Geometry check sheet. Reference: the model listing, model coordinates, mm. A direction names the side the tool comes from. Give positions to 0.01 mm unless a question says otherwise; leave off trailing zeros. Loops run counter-clockwise (first coordinate to the right, second up) from the corner with the lowest first, then second, coordinate; pieces in that order, holes last.
Autodesk Inventor part; units mm, degrees
ref_plane "Work Plane1" through (50.664548, -102.160446, 0.616313) normal (0, -0.9659258, -0.258819) x (1, 0, 0)
ref_plane "YZ Plane" through (0, 0, 0) normal (1, 0, 0) x (0, 1, 0)
ref_plane "XZ Plane" through (0, 0, 0) normal (0, 1, 0) x (-1, 0, 0)
sketch "Sketch1" plane through (0, 0, 0) normal (0, 0, 1) x (1, 0, 0)
  line L0 (-10.454202, 14.601943) -> (210.208298, 14.601943)
  line L1 (216.558298, 8.251943) -> (216.558298, -98.110557)
  line L2 (210.208298, -104.460557) -> (-10.454202, -104.460557)
  line L3 (-16.804202, -98.110557) -> (-16.804202, 8.251943)
  line L4 (99.877048, 12.220693) -> (-10.454202, 12.220693)
  line L5 (-14.422952, 8.251943) -> (-14.422952, -44.929307)
  line L6 (99.877048, 12.220693) -> (210.208298, 12.220693)
  line L7 (214.177048, 8.251943) -> (214.177048, -44.929307)
  line L8 (99.877048, -102.079307) -> (210.208298, -102.079307)
  line L9 (214.177048, -98.110557) -> (214.177048, -44.929307)
  line L10 (99.877048, -102.079307) -> (-10.454202, -102.079307)
  line L11 (-14.422952, -98.110557) -> (-14.422952, -44.929307)
  arc A0 (-10.454202, 14.601943) -> (-16.804202, 8.251943) centre (-10.454202, 8.251943) ccw
  arc A1 (216.558298, 8.251943) -> (210.208298, 14.601943) centre (210.208298, 8.251943) ccw
  arc A2 (210.208298, -104.460557) -> (216.558298, -98.110557) centre (210.208298, -98.110557) ccw
  arc A3 (-16.804202, -98.110557) -> (-10.454202, -104.460557) centre (-10.454202, -98.110557) ccw
  arc A4 (-10.454202, 12.220693) -> (-14.422952, 8.251943) centre (-10.454202, 8.251943) ccw
  arc A5 (214.177048, 8.251943) -> (210.208298, 12.220693) centre (210.208298, 8.251943) ccw
  arc A6 (210.208298, -102.079307) -> (214.177048, -98.110557) centre (210.208298, -98.110557) ccw
  arc A7 (-14.422952, -98.110557) -> (-10.454202, -102.079307) centre (-10.454202, -98.110557) ccw
  point P0 (0, 0)
  point P1 (-16.804202, 14.601943)
  point P2 (216.558298, -104.460557)
  point P3 (216.558298, 14.601943)
  point P4 (-16.804202, -104.460557)
  dimension "d0" = 233.3625
  dimension "d1" = 119.0625
  dimension "d9" = 6.35
  dimension "d10" = 3.96875
extrude "Extrusion1" add sketch "Sketch1" along normal blind 2.38125 contours L0 A1 L1 A2 L2 A3 L3 A0 | L6 A5 L7 L9 A6 L8 L10 A7 L11 L5 A4 L4
sketch "Sketch2" plane through (0, 0, 2.38125) normal (0, 0, 1) x (1, 0, 0)
  line L0 (210.208298, 14.601943) -> (-10.454202, 14.601943)
  arc A0 (-10.454202, 14.601943) -> (-16.804202, 8.251943) centre (-10.454202, 8.251943) ccw
  line L1 (-16.804202, 8.251943) -> (-16.804202, -98.110557)
  arc A1 (-16.804202, -98.110557) -> (-10.454202, -104.460557) centre (-10.454202, -98.110557) ccw
  line L2 (-10.454202, -104.460557) -> (210.208298, -104.460557)
  arc A2 (210.208298, -104.460557) -> (216.558298, -98.110557) centre (210.208298, -98.110557) ccw
  line L3 (216.558298, -98.110557) -> (216.558298, 8.251943)
  arc A3 (216.558298, 8.251943) -> (210.208298, 14.601943) centre (210.208298, 8.251943) ccw
  line L4 (99.877048, 12.220693) -> (-10.454202, 12.220693)
  line L5 (-14.422952, 8.251943) -> (-14.422952, -44.929307)
  line L6 (99.877048, -102.079307) -> (-10.454202, -102.079307)
  line L7 (-14.422952, -98.110557) -> (-14.422952, -44.929307)
  line L8 (99.877048, -102.079307) -> (210.208298, -102.079307)
  line L9 (214.177048, -98.110557) -> (214.177048, -44.929307)
  line L10 (99.877048, 12.220693) -> (210.208298, 12.220693)
  line L11 (214.177048, 8.251943) -> (214.177048, -44.929307)
  arc A4 (-10.454202, 12.220693) -> (-14.422952, 8.251943) centre (-10.454202, 8.251943) ccw
  arc A5 (214.177048, 8.251943) -> (210.208298, 12.220693) centre (210.208298, 8.251943) ccw
  arc A6 (210.208298, -102.079307) -> (214.177048, -98.110557) centre (210.208298, -98.110557) ccw
  arc A7 (-14.422952, -98.110557) -> (-10.454202, -102.079307) centre (-10.454202, -98.110557) ccw
  point P0 (0, 0)
  dimension "d15" = 3.96875
extrude "Extrusion2" add sketch "Sketch2" along normal blind 2.38125
sketch "Sketch3" plane through (0, 0, 4.7625) normal (0, 0, 1) x (1, 0, 0)
  arc A0 (-10.454202, 12.220693) -> (-14.422952, 8.251943) centre (-10.454202, 8.251943) ccw
  line L0 (-10.454202, 12.220693) -> (210.208298, 12.220693)
  arc A1 (214.177048, 8.251943) -> (210.208298, 12.220693) centre (210.208298, 8.251943) ccw
  line L1 (214.177048, 8.251943) -> (214.177048, -98.110557)
  arc A2 (210.208298, -102.079307) -> (214.177048, -98.110557) centre (210.208298, -98.110557) ccw
  line L2 (210.208298, -102.079307) -> (-10.454202, -102.079307)
  arc A3 (-14.422952, -98.110557) -> (-10.454202, -102.079307) centre (-10.454202, -98.110557) ccw
  line L3 (-14.422952, -98.110557) -> (-14.422952, 8.251943)
  line L4 (210.208298, 14.601943) -> (-10.454202, 14.601943)
  arc A4 (-10.454202, 14.601943) -> (-16.804202, 8.251943) centre (-10.454202, 8.251943) ccw
  line L5 (-16.804202, 8.251943) -> (-16.804202, -98.110557)
  arc A5 (-16.804202, -98.110557) -> (-10.454202, -104.460557) centre (-10.454202, -98.110557) ccw
  line L6 (-10.454202, -104.460557) -> (210.208298, -104.460557)
  arc A6 (210.208298, -104.460557) -> (216.558298, -98.110557) centre (210.208298, -98.110557) ccw
  line L7 (216.558298, -98.110557) -> (216.558298, 8.251943)
  arc A7 (216.558298, 8.251943) -> (210.208298, 14.601943) centre (210.208298, 8.251943) ccw
  line L8 (214.177048, -44.929307) -> (214.177048, -41.754307)
  line L9 (214.177048, -41.754307) -> (216.558298, -41.754307)
  line L10 (216.558298, -41.754307) -> (216.558298, -44.929307)
  line L11 (216.558298, -44.929307) -> (216.558298, -48.104307)
  line L12 (216.558298, -48.104307) -> (214.177048, -48.104307)
  line L13 (214.177048, -48.104307) -> (214.177048, -44.929307)
  line L14 (-14.422952, -44.929307) -> (-14.422952, -41.754307)
  line L15 (-14.422952, -41.754307) -> (-16.804202, -41.754307)
  line L16 (-16.804202, -41.754307) -> (-16.804202, -44.929307)
  line L17 (-16.804202, -44.929307) -> (-16.804202, -48.104307)
  line L18 (-16.804202, -48.104307) -> (-14.422952, -48.104307)
  line L19 (-14.422952, -48.104307) -> (-14.422952, -44.929307)
  point P0 (0, 0)
  dimension "d18" = 3.175
  dimension "d19" = 3.175
  dimension "d20" = 3.175
  dimension "d21" = 3.175
extrude "Extrusion3" add sketch "Sketch3" along normal blind 10.31875 contours A0 L3 L15 L5 A4 L4 A7 L7 L9 L1 A1 L0 | L3 A3 L2 A2 L1 L12 L7 A6 L6 A5 L5 L18
sketch "Sketch4" plane through (0, 0, 15.08125) normal (0, 0, 1) x (1, 0, 0)
  line L0 (214.177048, -41.754307) -> (216.558298, -41.754307)
  line L1 (216.558298, -41.754307) -> (216.558298, -48.104307)
  line L2 (216.558298, -48.104307) -> (214.177048, -48.104307)
  line L3 (214.177048, -48.104307) -> (214.177048, -41.754307)
  line L4 (-16.804202, -41.754307) -> (-14.422952, -41.754307)
  line L5 (-14.422952, -41.754307) -> (-14.422952, -48.104307)
  line L6 (-14.422952, -48.104307) -> (-16.804202, -48.104307)
  line L7 (-16.804202, -48.104307) -> (-16.804202, -41.754307)
  point P0 (0, 0)
  dimension "d24" = 2.38125
  dimension "d25" = 6.35
  dimension "d26" = 2.38125
  dimension "d27" = 6.35
extrude "Extrusion4" add sketch "Sketch4" against normal blind 7.9375
sketch "Sketch5" plane through (0, 0, 0) normal (0, 0, -1) x (-1, 0, 0)
  arc A0 (-210.208298, 14.601943) -> (-216.558298, 8.251943) centre (-210.208298, 8.251943) ccw
  line L0 (-210.208298, 8.251943) -> (-99.877048, 8.251943)
  line L1 (-99.877048, 8.251943) -> (-99.877048, -44.929307)
  line L2 (-99.877048, -44.929307) -> (-210.208298, -44.929307)
  line L3 (-210.208298, -44.929307) -> (-210.208298, 8.251943)
  point P0 (0, 0)
hole "Hole1" at (99.877048, -44.929307, 0) direction (0, 0, 1) diameter 19.05 end through all
sketch "Sketch7" plane through (-10.454202, -104.460557, 0) normal (0, -1, 0) x (1, 0, 0)
  line L0 (220.6625, 0) -> (0, 0)
  line L1 (0, 15.08125) -> (220.6625, 15.08125)
  line L2 (61.11875, 15.08125) -> (61.11875, 0)
  line L3 (159.54375, 15.08125) -> (159.54375, 0)
  line L4 (61.11875, 15.08125) -> (159.54375, 15.08125)
  line L5 (159.54375, 0) -> (61.11875, 0)
  point P0 (10.454202, 0)
extrude "Extrusion5" add sketch "Sketch7" along normal blind 25.4
sketch "Sketch8" plane through (149.089548, -104.460557, 15.08125) normal (1, 0, 0) x (0, 0, -1)
  line L0 (15.08125, 0) -> (-19.502452, -9.266675)
  line L1 (15.08125, 0) -> (50.884933, 0) construction
  point P0 (15.08125, 104.460557)
  dimension "d41" = 165
split body "Split1" sketch "Sketch8" result one side removed curves L0 removed pieces at (116.281215, -121.39389, 0.5)
ref_plane "Work Plane1" through (50.664548, -102.160446, 0.616313) normal (0, -0.9659258, -0.258819) x (1, 0, 0)
sketch "Sketch10" plane through (0, 0, 15.08125) normal (0, 0, 1) x (1, 0, 0)
  line L0 (99.877048, -104.460557) -> (111.307048, -104.460557)
  line L1 (111.307048, -104.460557) -> (111.307048, -108.501565)
  line L2 (99.877048, -104.460557) -> (88.447048, -104.460557)
  line L3 (88.447048, -104.460557) -> (88.447048, -108.501565)
  line L4 (88.447048, -108.501565) -> (111.307048, -108.501565)
  point P0 (0, 0)
  dimension "d43" = 11.43
  dimension "d44" = 11.43
split body "Split2" sketch "Sketch10" result one side removed curves L4 L1 L0 L2 L3 removed pieces at (99.877048, -106.671599, 10.183576)
sketch "Sketch13" plane through (50.664548, -102.160446, 0.616313) normal (0, -0.9659258, -0.258819) x (1, 0, 0)
  line L0 (37.7825, 0) -> (37.7825, 15.613259)
  line L1 (0, 15.613259) -> (37.7825, 15.613259)
  line L2 (0, 0) -> (0, 15.613259)
  line L3 (37.7825, 0) -> (0, 0)
  line L4 (60.6425, 15.613259) -> (60.6425, 0)
  line L5 (98.425, 0) -> (60.6425, 0)
  line L6 (98.425, 15.613259) -> (98.425, 0)
  line L7 (60.6425, 15.613259) -> (98.425, 15.613259)
  line L8 (0, 15.613259) -> (98.425, 15.613259)
  line L9 (49.2125, 15.613259) -> (49.2125, 0)
  line L10 (49.2125, 7.806629) -> (32.8295, 7.806629)
  line L11 (49.2125, 7.806629) -> (65.5955, 7.806629)
  line L12 (65.5955, 7.806629) -> (80.0735, 7.806629)
  line L13 (32.8295, 7.806629) -> (18.3515, 7.806629)
  point P0 (-50.664548, -27.036381)
  dimension "d45" = 16.383
  dimension "d46" = 16.383
  dimension "d47" = 14.478
  dimension "d48" = 14.478
hole "Hole2" at (69.016048, -104.18095, 8.156938) at (116.260048, -104.18095, 8.156938) at (83.494048, -104.18095, 8.156938) at (130.738048, -104.18095, 8.156938) direction (0, 0.9659258, 0.258819) diameter 6.35 end through all
sketch "Sketch14" plane through (50.664548, -102.160446, 0.616313) normal (0, -0.9659258, -0.258819) x (1, 0, 0)
  line L0 (37.7825, 0) -> (37.7825, 15.613259)
  line L1 (0, 15.613259) -> (37.7825, 15.613259)
  line L2 (0, 0) -> (0, 15.613259)
  line L3 (37.7825, 0) -> (0, 0)
  line L4 (60.6425, 15.613259) -> (60.6425, 0)
  line L5 (98.425, 0) -> (60.6425, 0)
  line L6 (98.425, 15.613259) -> (98.425, 0)
  line L7 (60.6425, 15.613259) -> (98.425, 15.613259)
  line L8 (0, 15.613259) -> (98.425, 15.613259)
  line L9 (49.2125, 15.613259) -> (49.2125, 0)
  line L10 (49.2125, 7.806629) -> (65.5955, 7.806629)
  line L11 (65.5955, 7.806629) -> (80.0735, 7.806629)
  line L12 (49.2125, 7.806629) -> (32.8295, 7.806629)
  line L13 (32.8295, 7.806629) -> (18.3515, 7.806629)
  point P0 (-50.664548, -27.036381)
  dimension "d56" = 16.383
  dimension "d57" = 14.478
  dimension "d58" = 16.383
  dimension "d59" = 14.478
hole "Hole3" at (69.016048, -104.18095, 8.156938) at (83.494048, -104.18095, 8.156938) at (116.260048, -104.18095, 8.156938) at (130.738048, -104.18095, 8.156938) direction (0, -0.9659258, -0.258819) diameter 3.175 end through all
sketch "Sketch15" plane through (0, 0, 4.7625) normal (0, 0, 1) x (1, 0, 0)
  line L0 (216.558298, -41.754307) -> (214.177048, -41.754307)
  line L1 (214.177048, -41.754307) -> (214.177048, -48.104307)
  line L2 (216.558298, -41.754307) -> (214.177048, -41.754307)
  line L3 (214.177048, -41.754307) -> (214.177048, -48.104307)
  line L4 (214.177048, -48.104307) -> (216.558298, -48.104307)
  line L5 (216.558298, -48.104307) -> (216.558298, -41.754307)
  point P0 (0, 0)
extrude "Extrusion6" add sketch "Sketch15" along normal blind 2.3876
sketch "Sketch16" plane through (0, 0, 4.7625) normal (0, 0, 1) x (1, 0, 0)
  line L0 (-14.422952, -41.754307) -> (-16.804202, -41.754307)
  line L1 (-16.804202, -41.754307) -> (-16.804202, -48.104307)
  line L2 (-14.422952, -41.754307) -> (-16.804202, -41.754307)
  line L3 (-16.804202, -41.754307) -> (-16.804202, -48.104307)
  line L4 (-16.804202, -48.104307) -> (-14.422952, -48.104307)
  line L5 (-14.422952, -48.104307) -> (-14.422952, -41.754307)
  point P0 (0, 0)
extrude "Extrusion7" add sketch "Sketch16" along normal blind 2.3876
sketch "Sketch17" plane through (0, 0, 0) normal (0, 0, -1) x (-1, 0, 0)
  arc A0 (10.454202, -104.460557) -> (16.804202, -98.110557) centre (10.454202, -98.110557) ccw
  arc A1 (16.804202, 8.251943) -> (10.454202, 14.601943) centre (10.454202, 8.251943) ccw
  arc A2 (-210.208298, 14.601943) -> (-216.558298, 8.251943) centre (-210.208298, 8.251943) ccw
  arc A3 (-216.558298, -98.110557) -> (-210.208298, -104.460557) centre (-210.208298, -98.110557) ccw
  point P0 (0, 0)
hole "Hole4" at (210.208298, 8.251943, 0) at (-10.454202, 8.251943, 0) at (-10.454202, -98.110557, 0) at (210.208298, -98.110557, 0) direction (0, 0, 1) diameter 3.175 end through all
properties part number "Master Tablet Enclosure"
1) Sectioned sample at A-A on x = 16.5. Enter the section's corners in (y, z).
2) Sectioned sample at C-C on y = -39.5. Enter the section's corners in (x, z).
3) Depth check by flat-ended pin: P1, Ø1, axis at x = 38, y = -61, coming from the +Z side; P2, Ø1.5, axis at x = 48.5, z = 7.5, coming from the -Y side; P3, Ø2.5, axis at x = 210.21, y = 8.25, coming from the +Z side; P4, Ø2, axis at y = -106.5, z = 5, coming from the +X side. Enter the tip coordinate at first touch or a pass-through.
4) Sectioned sample at D-D on y = -52. Enter the section's corners in (x, z).
5) Tool access check on faces 5 (the flat face through (20, -104.461, 7)), 6 (the flat face through (132.1, -103.83, 6.84)), 7 (the flat face through (149.09, -106, 9)), 8 (the flat face through (88.447, -106, 11)). Record the directions out of +Z, -Z, +X, -X, +Y, -Y that give a thin tool (end or side, any length) a straight path to the whole face; none if there is none.
6) Scan lines: line 1 along Y through (x, z) = (151.5, 11.5); line 2 along X through (y, z) = (-79, 3.75); line 3 along Z through (x, y) = (73, -36). Record each from-to range of solid material in increasing order.
7) Mould release check, pull along Y, two halves, no side actions. Record for faces 1 (the flat face through (179, -104.461, 7)), 2 (the flat face through (98, -57, 2.381)), 3 (the cylindrical face through (-13.23, -100.948, 8.642)), 4 (the flat face through (-16.804, -44, 7)): +Y half, -Y half, draft (parallel to the pull), parting line (faces both ways), or undercut.
8) Sectioned sample at B-B on y = -27. Enter the section's corners in (x, z), plus the area to 3 significant figures.
Determined:
1. outline: (-104.46, 0) - (14.6, 0) - (14.6, 15.08) - (12.22, 15.08) - (12.22, 2.38) - (-102.08, 2.38) - (-102.08, 15.08) - (-104.46, 15.08) - close
2. outline: (-16.8, 0) - (92.05, 0) - (92.05, 2.38) - (-14.42, 2.38) - (-14.42, 15.08) - (-16.8, 15.08) - close; (107.7, 0) - (216.56, 0) - (216.56, 15.08) - (214.18, 15.08) - (214.18, 2.38) - (107.7, 2.38) - close
3. P1: stops at z = 2.38
3. P2: stops at y = -104.46
3. P3: passes through
3. P4: stops at x = 149.09
4. outline: (-16.8, 0) - (93.49, 0) - (93.49, 2.38) - (-14.42, 2.38) - (-14.42, 15.08) - (-16.8, 15.08) - close; (106.26, 0) - (216.56, 0) - (216.56, 15.08) - (214.18, 15.08) - (214.18, 2.38) - (106.26, 2.38) - close
5. face 5: +Z, -Z, -X, -Y
5. face 6: none
5. face 7: +Z, -Z, +X, -Y
5. face 8: +Z, -Z, -Y
6. line 1: y = -104.46 to -102.08, 12.22 to 14.6
6. line 2: x = -16.8 to -14.42, 214.18 to 216.56
6. line 3: z = 0 to 2.38
7. face 1: -Y half
7. face 2: undercut
7. face 3: undercut
7. face 4: draft
8. outline: (-16.8, 0) - (216.56, 0) - (216.56, 15.08) - (214.18, 15.08) - (214.18, 2.38) - (-14.42, 2.38) - (-14.42, 15.08) - (-16.8, 15.08) - close
8. area: 616 mm2
